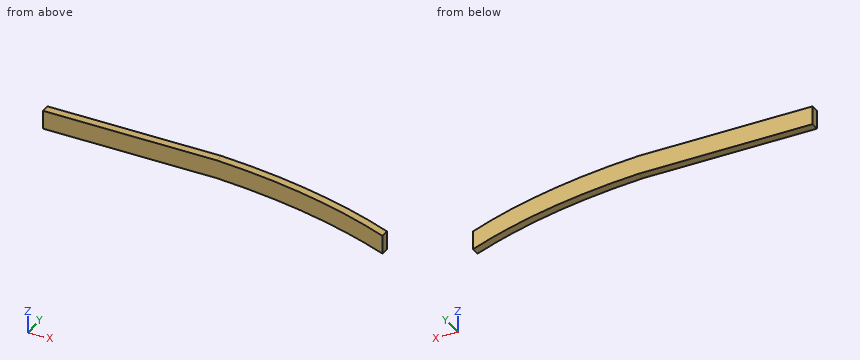
```python
from build123d import *

# Parameters (mm, degrees)
BOSS_EXTRUDE1_DEPTH = 3


with BuildPart() as part:
    # Sketch1 → Boss-Extrude1 (new body)
    with BuildSketch(Plane(origin=(0, 0, 0), x_dir=(1, 0, 0), z_dir=(0, 1, 0))):
        with BuildLine():
            Line((0, 0), (61.5, 0))
            add(Edge.make_bspline(
                [(61.5, 0), (96.079868576, 1.689945504), (120.026085552, 10.3)],
                knots=[0, 0, 0, 1, 1, 1], degree=2))
            Line((120.026085552, 10.3), (120.028762053, 16.803234674))
            add(Edge.make_bspline(
                [(61.5, 6.5), (96.082545077, 8.193180177), (120.028762053, 16.803234674)],
                knots=[0, 0, 0, 1, 1, 1], degree=2))
            Line((61.5, 6.5), (0, 6.5))
            Line((0, 6.5), (0, 0))
        make_face()
    extrude(amount=BOSS_EXTRUDE1_DEPTH)


solid = part.part
```
The listing builds one solid part. Answer for the finished solid, in the listing's coordinates (mm). Give positions to 0.01 mm unless a question says otherwise; leave off trailing zeros. Order: outer loops, then holes, each group sorted by start corner. A loop starts at its lowest first (then second) coordinate and runs counter-clockwise, first axis right, second up.
1) Find section A-A on x = 36. Write down the section's boundary in (y, z).
Reported:
outline: (0, -6.5) - (3, -6.5) - (3, 0) - (0, 0) - close
2) Consider line 1 along Z through (x, y) = (56, 2.6); line 2 along Z through (x, y) = (73, 1.35). Determine where each line is inside the solid, lowest interval first.
Reported:
line 1: z = -6.5 to 0
line 2: z = -7.28 to -0.78
3) Given P1, Ø1, axis at x = 103, y = 1.5, coming from the +Z side; P2, Ø0.9, axis at x = 22.5, y = 1.5, coming from the -Z side; P3, Ø1.5, axis at x = 90.5, y = 2, coming from the +Z side, each flat-ended and moving along its own axis, determine where each tip first touches the part or whether it passes through.
Reported:
P1: stops at z = -5.24
P2: stops at z = -6.5
P3: stops at z = -2.81
